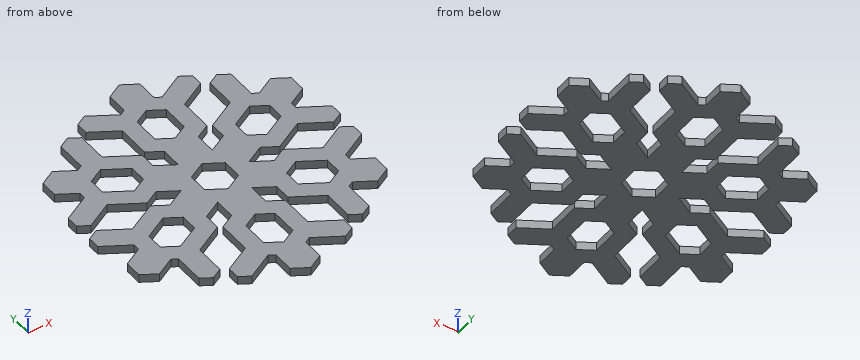
```python
from build123d import *

# Parameters (mm, degrees)
F1_DEPTH = 1.5
F2_SCALE = 2


with BuildPart() as f1:
    # F0 (on Top) → F1 (new body)
    with BuildSketch(Plane.XY):
        Polygon((-6.1687498137, 0), (-3.0843749069, 1.7807646828), (-3.0843749069, 5.3422940483), (-6.3761018887, 7.2427735073), (-6.3761018887, 10.2092925487), (-11.6322247993, 13.243916526), (-13.537250454, 14.3437836005), (-15.4422761086, 13.243916526), (-16.480613925, 12.6444319082), (-19.1907062114, 11.0797593971), (-19.1907062114, 7.9504143749), (-19.1907062114, 6.7514451393), (-19.1907062114, 4.5517109903), (-17.2856805568, 3.4518439158), (-12.0295576462, 0.4172199384), (-9.4604767956, 1.9004794591), align=None)
        Polygon((-16.1907062114, 6.2837617978), (-16.1907062114, 9.3477085895), (-13.537250454, 10.8796819854), (-9.3761018887, 8.4772417411), (-9.3761018887, 5.4132949494), (-12.0295576462, 3.8813215535), align=None, mode=Mode.SUBTRACT)
        Polygon((-3.0843749069, -1.7807646828), (-3.0843749069, 1.7807646828), (-6.1687498137, 0), align=None)
        Polygon((-3.0843749069, 5.3422940483), (-3.0843749069, 1.7807646828), (0, 3.5615293655), align=None)
        Polygon((-3.0843749069, 9.1432529664), (-3.0843749069, 5.3422940483), (0, 3.5615293655), (3.0843749069, 5.3422940483), (3.0843749069, 9.1432529664), (5.6534557575, 10.6265124871), (5.6534557575, 16.6957604418), (5.6534557575, 18.8954945908), (3.7484301028, 19.9953616653), (2.7100922865, 20.5948462831), (0, 22.1595187942), (-2.7100922865, 20.5948462831), (-3.7484301028, 19.9953616653), (-5.6534557575, 18.8954945908), (-5.6534557575, 16.6957604418), (-5.6534557575, 10.6265124871), align=None)
        Polygon((-2.6534557575, 17.1634437832), (0, 18.6954171791), (2.6534557575, 17.1634437832), (2.6534557575, 12.3585632946), (0, 10.8265898988), (-2.6534557575, 12.3585632946), align=None, mode=Mode.SUBTRACT)
        Polygon((-3.0843749069, -1.7807646828), (-6.1687498137, 0), (-9.4604767956, -1.9004794591), (-12.0295576462, -0.4172199384), (-17.2856805568, -3.4518439158), (-19.1907062114, -4.5517109903), (-19.1907062114, -6.7514451393), (-19.1907062114, -7.9504143749), (-19.1907062114, -11.0797593971), (-16.480613925, -12.6444319082), (-15.4422761086, -13.243916526), (-13.537250454, -14.3437836005), (-11.6322247993, -13.243916526), (-6.3761018887, -10.2092925487), (-6.3761018887, -7.2427735073), (-3.0843749069, -5.3422940483), align=None)
        Polygon((-13.537250454, -10.8796819854), (-16.1907062114, -9.3477085895), (-16.1907062114, -6.2837617978), (-12.0295576462, -3.8813215535), (-9.3761018887, -5.4132949494), (-9.3761018887, -8.4772417411), align=None, mode=Mode.SUBTRACT)
        Polygon((3.0843749069, 5.3422940483), (0, 3.5615293655), (3.0843749069, 1.7807646828), align=None)
        Polygon((0, -3.5615293655), (-3.0843749069, -1.7807646828), (-3.0843749069, -5.3422940483), align=None)
        Polygon((6.3761018887, 7.2427735073), (3.0843749069, 5.3422940483), (3.0843749069, 1.7807646828), (6.1687498137, 0), (9.4604767956, 1.9004794591), (12.0295576462, 0.4172199384), (17.2856805568, 3.4518439158), (19.1907062114, 4.5517109903), (19.1907062114, 6.7514451393), (19.1907062114, 7.9504143749), (19.1907062114, 11.0797593971), (16.480613925, 12.6444319082), (15.4422761086, 13.243916526), (13.537250454, 14.3437836005), (11.6322247993, 13.243916526), (6.3761018887, 10.2092925487), align=None)
        Polygon((13.537250454, 10.8796819854), (16.1907062114, 9.3477085895), (16.1907062114, 6.2837617978), (12.0295576462, 3.8813215535), (9.3761018887, 5.4132949494), (9.3761018887, 8.4772417411), align=None, mode=Mode.SUBTRACT)
        Polygon((6.1687498137, 0), (3.0843749069, 1.7807646828), (3.0843749069, -1.7807646828), align=None)
        Polygon((0, -3.5615293655), (-3.0843749069, -5.3422940483), (-3.0843749069, -9.1432529664), (-5.6534557575, -10.6265124871), (-5.6534557575, -16.6957604418), (-5.6534557575, -18.8954945908), (-3.7484301028, -19.9953616653), (-2.7100922865, -20.5948462831), (0, -22.1595187942), (2.7100922865, -20.5948462831), (3.7484301028, -19.9953616653), (5.6534557575, -18.8954945908), (5.6534557575, -16.6957604418), (5.6534557575, -10.6265124871), (3.0843749069, -9.1432529664), (3.0843749069, -5.3422940483), align=None)
        Polygon((2.6534557575, -17.1634437832), (0, -18.6954171791), (-2.6534557575, -17.1634437832), (-2.6534557575, -12.3585632946), (0, -10.8265898988), (2.6534557575, -12.3585632946), align=None, mode=Mode.SUBTRACT)
        Polygon((3.0843749069, -1.7807646828), (0, -3.5615293655), (3.0843749069, -5.3422940483), align=None)
        Polygon((9.4604767956, -1.9004794591), (6.1687498137, 0), (3.0843749069, -1.7807646828), (3.0843749069, -5.3422940483), (6.3761018887, -7.2427735073), (6.3761018887, -10.2092925487), (11.6322247993, -13.243916526), (13.537250454, -14.3437836005), (15.4422761086, -13.243916526), (16.480613925, -12.6444319082), (19.1907062114, -11.0797593971), (19.1907062114, -7.9504143749), (19.1907062114, -6.7514451393), (19.1907062114, -4.5517109903), (17.2856805568, -3.4518439158), (12.0295576462, -0.4172199384), align=None)
        Polygon((16.1907062114, -6.2837617978), (16.1907062114, -9.3477085895), (13.537250454, -10.8796819854), (9.3761018887, -8.4772417411), (9.3761018887, -5.4132949494), (12.0295576462, -3.8813215535), align=None, mode=Mode.SUBTRACT)
        Polygon((-10.4125291109, 19.4434127235), (-5.6534557575, 16.6957604418), (-5.6534557575, 18.8954945908), (-3.7484301028, 19.9953616653), (-8.5075034563, 22.743013947), (-10.4125291109, 21.6431468725), align=None)
        Polygon((-13.537250454, 14.3437836005), (-11.6322247993, 13.243916526), (-11.6322247993, 18.7392210894), (-13.537250454, 19.839088164), (-15.4422761086, 18.7392210894), (-15.4422761086, 13.243916526), align=None)
        Polygon((-22.0447539102, 0.704191634), (-17.2856805568, 3.4518439158), (-19.1907062114, 4.5517109903), (-19.1907062114, 6.7514451393), (-23.9497795649, 4.0037928576), (-23.9497795649, 1.8040587086), align=None)
        Polygon((-19.1907062114, -4.5517109903), (-17.2856805568, -3.4518439158), (-22.0447539102, -0.704191634), (-23.9497795649, -1.8040587086), (-23.9497795649, -4.0037928576), (-19.1907062114, -6.7514451393), align=None)
        Polygon((5.6534557575, 18.8954945908), (5.6534557575, 16.6957604418), (10.4125291109, 19.4434127235), (10.4125291109, 21.6431468725), (8.5075034563, 22.743013947), (3.7484301028, 19.9953616653), align=None)
        Polygon((11.6322247993, 18.7392210894), (11.6322247993, 13.243916526), (13.537250454, 14.3437836005), (15.4422761086, 13.243916526), (15.4422761086, 18.7392210894), (13.537250454, 19.839088164), align=None)
        Polygon((-11.6322247993, -18.7392210894), (-11.6322247993, -13.243916526), (-13.537250454, -14.3437836005), (-15.4422761086, -13.243916526), (-15.4422761086, -18.7392210894), (-13.537250454, -19.839088164), align=None)
        Polygon((-5.6534557575, -18.8954945908), (-5.6534557575, -16.6957604418), (-10.4125291109, -19.4434127235), (-10.4125291109, -21.6431468725), (-8.5075034563, -22.743013947), (-3.7484301028, -19.9953616653), align=None)
        Polygon((22.0447539102, -0.704191634), (17.2856805568, -3.4518439158), (19.1907062114, -4.5517109903), (19.1907062114, -6.7514451393), (23.9497795649, -4.0037928576), (23.9497795649, -1.8040587086), align=None)
        Polygon((19.1907062114, 4.5517109903), (17.2856805568, 3.4518439158), (22.0447539102, 0.704191634), (23.9497795649, 1.8040587086), (23.9497795649, 4.0037928576), (19.1907062114, 6.7514451393), align=None)
        Polygon((10.4125291109, -19.4434127235), (5.6534557575, -16.6957604418), (5.6534557575, -18.8954945908), (3.7484301028, -19.9953616653), (8.5075034563, -22.743013947), (10.4125291109, -21.6431468725), align=None)
        Polygon((13.537250454, -14.3437836005), (11.6322247993, -13.243916526), (11.6322247993, -18.7392210894), (13.537250454, -19.839088164), (15.4422761086, -18.7392210894), (15.4422761086, -13.243916526), align=None)
        Polygon((-2.7100922865, 24.4353274889), (-2.7100922865, 20.5948462831), (0, 22.1595187942), (2.7100922865, 20.5948462831), (2.7100922865, 24.4353274889), (0, 26), align=None)
        Polygon((-19.1907062114, 11.0797593971), (-16.480613925, 12.6444319082), (-19.8065682119, 14.5646725111), (-22.5166604984, 13), (-22.5166604984, 9.8706549778), (-19.1907062114, 7.9504143749), align=None)
        Polygon((-19.1907062114, -11.0797593971), (-19.1907062114, -7.9504143749), (-22.5166604984, -9.8706549778), (-22.5166604984, -13), (-19.8065682119, -14.5646725111), (-16.480613925, -12.6444319082), align=None)
        Polygon((19.8065682119, 14.5646725111), (16.480613925, 12.6444319082), (19.1907062114, 11.0797593971), (19.1907062114, 7.9504143749), (22.5166604984, 9.8706549778), (22.5166604984, 13), align=None)
        Polygon((0, -22.1595187942), (-2.7100922865, -20.5948462831), (-2.7100922865, -24.4353274889), (0, -26), (2.7100922865, -24.4353274889), (2.7100922865, -20.5948462831), align=None)
        Polygon((22.5166604984, -9.8706549778), (19.1907062114, -7.9504143749), (19.1907062114, -11.0797593971), (16.480613925, -12.6444319082), (19.8065682119, -14.5646725111), (22.5166604984, -13), align=None)
    extrude(amount=F1_DEPTH)


with BuildPart() as f1_1:
    # F2: moved
    add(f1.part.scale(F2_SCALE))


solid = f1_1.part
```
Check sheet for the modelled part. Datum: model origin and axes. Units: mm. Coordinates: 2 decimals unless noted, no trailing zeros. Write each loop counter-clockwise with the first axis right and the second up, starting at its lowest first coordinate (ties: lowest second). Pieces come first, ordered by that corner, then holes. Notation, with made-up numbers: M 51,18 L 56,18 A20 ccw 56,43 Z; hole C 16,85.25 d4. An arc over 180 degrees is marked long. Write item = value, one per line. Start each with the question number.
1. Sectioned sample at B-B (x = 9). Record the cut outline in (y, z).
2. Go/stop test with flat-tipped pins: pin 1 (1.5 mm diameter, centred on y = 41.5, z = 2, fed in from -X); pin 2 (1.5 mm diameter, centred on y = -24.5, z = 1, fed in from +X); pin 3 (0.9 mm diameter, centred on y = 31, z = 1, fed in from +X). Record where each tip stops, or that it passes through.
3. Thickness scan on probe 1 along X at (y, z) = (33, 0.55); probe 2 along Y at (x, z) = (0, 0.45); probe 3 along Y at (x, z) = (18.5, 1.3). Record the ranges inside material, lowest first.
4. Sectioned sample at A-A (y = -31). Record the cut outline in (x, z).
5. Sectioned sample at C-C (z = 1.4). State how many separate pieces and enclosed holes the cut face has, then the cut area to 3 significant figures.
6. Sectioned sample at D-D (x = -29). Record the cut outline in (y, z), then the cut area to 3 significant figures.
The answers:
q1.outline = M -40.86,0 L -19.92,0 L -19.92,3 L -40.86,3 Z; M -12.32,0 L 12.32,0 L 12.32,3 L -12.32,3 Z; M 19.92,0 L 40.86,0 L 40.86,3 L 19.92,3 Z
q2.pin_1 = -20.83
q2.pin_2 = 45.03
q2.pin_3 = 30.88
q3.probe_1 = -30.88 to -23.26, -11.31 to -5.31, 5.31 to 11.31, 23.26 to 30.88
q3.probe_2 = -52 to -37.39, -21.65 to -7.12, 7.12 to 21.65, 37.39 to 52
q3.probe_3 = -44.63 to -37.54, -23.74 to -3.56, 3.56 to 23.74, 37.54 to 44.63
q4.outline = M -30.88,0 L -23.26,0 L -23.26,3 L -30.88,3 Z; M -11.31,0 L -5.31,0 L -5.31,3 L -11.31,3 Z; M 5.31,0 L 11.31,0 L 11.31,3 L 5.31,3 Z; M 23.26,0 L 30.88,0 L 30.88,3 L 23.26,3 Z
q5.separate_pieces = 1
q5.enclosed_holes = 7
q5.area = 4,520 mm²
q6.outline = M -38.57,0 L -20.65,0 L -20.65,3 L -38.57,3 Z; M -10.62,0 L -3.69,0 L -3.69,3 L -10.62,3 Z; M 3.69,0 L 10.62,0 L 10.62,3 L 3.69,3 Z; M 20.65,0 L 38.57,0 L 38.57,3 L 20.65,3 Z
q6.area = 149 mm²
